Verification items for the finished model (mm, model axes). Face numbers are marked on the shaded views. A direction names the side the tool comes from. Give positions to 0.01 mm unless a question says otherwise; leave off trailing zeros. Order: outer loops, then holes, each group sorted by start corner. A loop starts at its lowest first (then second) coordinate and runs counter-clockwise, first axis right, second up.
(1) Scan lines: L1, parallel to Y at x = 20.5, z = 14.75; L2, parallel to X at y = -14.5, z = 13.5; L3, parallel to X at y = 0.5, z = 9.25. Record each from-to range of solid material in increasing order.
(2) Sectioned sample at D-D on x = 12.5. Record the cut outline in (y, z).
(3) Access from +Z, -Z, +X, -X, +Y, -Y to the whole of each face (thin tool, end or side, straight path). Record for the marked faces 4, 5, 6 and 7.
(4) Sectioned sample at B-B on y = 12. Record the cut outline in (x, z), plus the area to 3 significant figures.
(5) Mould release check, pull along Y, two halves, no side actions. Record for the marked faces 1, 2 and 3: pulls with the +Y half, pulls with the -Y half, needs draft (parallel to the pull), parting line crosses it, or undercut.
(6) Gauge pin test, flat ends, axial feed: pin 1 (6 mm diameter, centred on x = -10, z = 22, fed in from +Y); pin 2 (21.5 mm diameter, centred on x = -12.5, y = 0, fed in from +Z); pin 3 (3 mm diameter, centred on x = -21.5, y = 12.5, fed in from +Z). Record the tip position at first contact, or that the pin passes through.
(7) Sectioned sample at C-C on y = 0. Record the cut outline in (x, z).
(8) Sectioned sample at A-A on z = 15.25. Record the cut outline in (x, y).
```python
from build123d import *

# Parameters (mm, degrees)
F6_W      = 50
F6_H      = 6
F7_DEPTH  = 30
F0_W      = 50
F0_H      = 30
F8_DEPTH  = 10
F1_W      = 6
F1_H      = 6
F2_W      = 6
F2_H      = 6
F11_DEPTH = 16
F13_R     = 3.125
F14_DEPTH = 10
F9_R      = 8.25
F15_DEPTH = 7
F10_R     = 8.25
F16_DEPTH = 10


with BuildPart() as f7:
    # F6 (on Top) → F7 (new body)
    with BuildSketch(Plane.XY):
        with Locations((0, -18)):
            Rectangle(F6_W, F6_H)
    extrude(amount=F7_DEPTH)

    # F0 (on Top) → F8 (join)
    with BuildSketch(Plane.XY):
        Rectangle(F0_W, F0_H)
    extrude(amount=F8_DEPTH)

    # F1 (on Top) + F2 (on Top) → F11 (join)
    with BuildSketch(Plane.XY):
        with Locations((-22, 12)):
            Rectangle(F1_W, F1_H)
    with BuildSketch(Plane.XY):
        with Locations((22, 12)):
            Rectangle(F2_W, F2_H)
        with Locations((22, -12)):
            Rectangle(F2_W, F2_H)
        with Locations((-22, -12)):
            Rectangle(F2_W, F2_H)
    extrude(amount=F11_DEPTH)

    # F13 (on face) → F14 (cut)
    with BuildSketch(Plane.XZ.offset(21)):
        with Locations((-12.3940734193, 24.9021667987)):
            Circle(F13_R)
        with Locations((12.5320926309, 25.2671018243)):
            Circle(F13_R)
    extrude(amount=-F14_DEPTH, mode=Mode.SUBTRACT)

    # F9 (on face) → F15 (cut)
    with BuildSketch(Plane.XY.offset(10)):
        with Locations((-12.5, 0)):
            Circle(F9_R)
    extrude(amount=-F15_DEPTH, mode=Mode.SUBTRACT)

    # F10 (on face) → F16 (cut)
    with BuildSketch(Plane.XY.offset(10)):
        with Locations((12.5, 0)):
            Circle(F10_R)
    extrude(amount=-F16_DEPTH, mode=Mode.SUBTRACT)


solid = f7.part
```
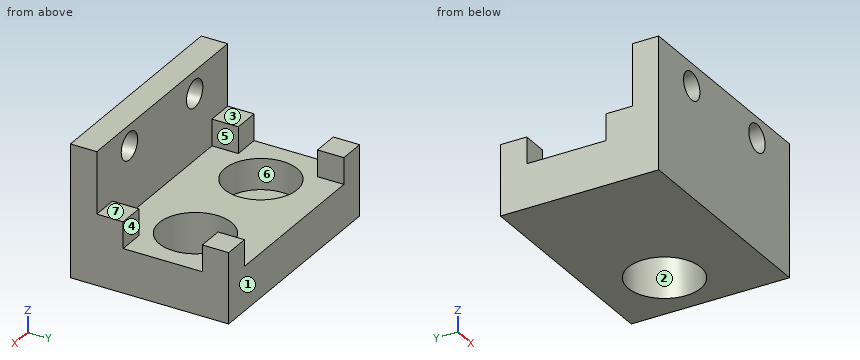
Ans:
1. L1: y = -21 to -9, 9 to 15
1. L2: x = -25 to -19, 19 to 25
1. L3: x = -25 to -20.73, -4.27 to 4.27, 20.73 to 25
2. outline: (-21, 0) - (-8.25, 0) - (-8.25, 10) - (-15, 10) - (-15, 22.14) - (-21, 22.14) - close; (-21, 28.39) - (-15, 28.39) - (-15, 30) - (-21, 30) - close; (8.25, 0) - (15, 0) - (15, 10) - (8.25, 10) - close
3. face 4: +Z, +X, -X
3. face 5: +Z, +Y
3. face 6: +Z
3. face 7: +Z, +X, -X, +Y
4. outline: (-25, 0) - (25, 0) - (25, 16) - (19, 16) - (19, 10) - (-19, 10) - (-19, 16) - (-25, 16) - close
4. area: 572 mm2
5. face 1: pulls with the +Y half
5. face 2: undercut
5. face 3: needs draft
6. pin 1: stops at y = -15
6. pin 2: stops at z = 10
6. pin 3: stops at z = 16
7. outline: (-25, 0) - (4.25, 0) - (4.25, 10) - (-4.25, 10) - (-4.25, 3) - (-20.75, 3) - (-20.75, 10) - (-25, 10) - close; (20.75, 0) - (25, 0) - (25, 10) - (20.75, 10) - close
8. outline: (-25, -21) - (25, -21) - (25, -9) - (19, -9) - (19, -15) - (-19, -15) - (-19, -9) - (-25, -9) - close; (-25, 9) - (-19, 9) - (-19, 15) - (-25, 15) - close; (19, 9) - (25, 9) - (25, 15) - (19, 15) - close
